```python
from build123d import *

# Parameters (mm, degrees)
SKETCH2_W           = 38.1
SKETCH2_H           = 304.8
SKETCH2_W_2         = 218.44
SKETCH2_H_2         = 38.1
BOSS_EXTRUDE1_DEPTH = 50.8
SKETCH4_W           = 228.6
SKETCH4_H           = 1.6002
CUT_EXTRUDE1_DEPTH  = 5.08


with BuildPart() as part:
    # Sketch2 → Boss-Extrude1 (new body)
    with BuildSketch(Plane(origin=(0, 0, 0), x_dir=(1, 0, 0), z_dir=(0, 1, 0))):
        with Locations((-128.27, 0)):
            Rectangle(SKETCH2_W, SKETCH2_H)
        with Locations((128.27, 0)):
            Rectangle(SKETCH2_W, SKETCH2_H)
        with Locations((0, -133.35)):
            Rectangle(SKETCH2_W_2, SKETCH2_H_2)
        with Locations((0, 133.35)):
            Rectangle(SKETCH2_W_2, SKETCH2_H_2)
    extrude(amount=BOSS_EXTRUDE1_DEPTH)

    # Sketch4 → Cut-Extrude1 (cut)
    with BuildSketch(Plane(origin=(-109.22, 0, 0), x_dir=(0, 0, -1), z_dir=(1, 0, 0))):
        with Locations((0, 37.2999)):
            Rectangle(SKETCH4_W, SKETCH4_H)
    cut_extrude1 = extrude(amount=-CUT_EXTRUDE1_DEPTH, mode=Mode.SUBTRACT)

    # Mirror1: Cut-Extrude1 across plane
    add(cut_extrude1.mirror(Plane(origin=(0, 0, 0), x_dir=(0, 0, 1), z_dir=(1, 0, 0))), mode=Mode.SUBTRACT)


solid = part.part
```
Could you check a few things on this model? Use its own coordinates, in mm. A direction names the side the tool comes from. Round coordinates to 2 decimals unless told otherwise and drop trailing zeros. Loops run counter-clockwise (first coordinate to the right, second up) from the corner with the lowest first, then second, coordinate; pieces in that order, holes last.
Q1. Thinking about a two-plate mould opening in X: for faces 1 (the flat face through (-109.22, 18, 2)), 2 (the flat face through (-133, 0, -2)), 3 (the flat face through (-147.32, 25, 2)), which applies, pulls with the +X half, pulls with the -X half, needs draft (parallel to the pull), parting line crosses it, or undercut?
Q2. On a 3-axis mill with a long thin cutter (end or side, diameter ignored), from which of +Z, -Z, +X, -X, +Y, -Y can I reach the whole of each face in a straight line? I mean faces 4 (the flat face through (-133, 50.8, -2)), 5 (the flat face through (109.22, 44, 2)). Say none if no direction works.
Q3. For P1, Ø5.5, axis at x = -112.5, z = -38.5, coming from the -Y side, with a flat end and sliding along its axis, tell me the tip position at first contact or that it passes through.
Q4. I want a section at A-A (x = 31.5). Write out the boundary of the cut face in (y, z), and give its area (3 significant figures).
Q5. I want a section at B-B (z = -36). Write out the boundary of the cut face in (x, y).
Q6. Please list where these lines run through material, in increasing order: L1, parallel to X at y = 14.5, z = -6; L2, parallel to Z at x = -105, y = 45.5; L3, parallel to Y at x = -110.5, z = 90.5.
Q7. I want a section at C-C (y = 28.5). Write out the boundary of the cut face in (x, z), and give its area (3 significant figures).
Answer below:
1. face 1: undercut
1. face 2: needs draft
1. face 3: pulls with the -X half
2. face 4: +Z, -Z, +X, -X, +Y
2. face 5: +Y, -Y
3. P1: stops at y = 0
4. outline: (0, -152.4) - (50.8, -152.4) - (50.8, -114.3) - (0, -114.3) - close; (0, 114.3) - (50.8, 114.3) - (50.8, 152.4) - (0, 152.4) - close
4. area: 3,870 mm2
5. outline: (-147.32, 0) - (-109.22, 0) - (-109.22, 36.5) - (-114.3, 36.5) - (-114.3, 38.1) - (-109.22, 38.1) - (-109.22, 50.8) - (-147.32, 50.8) - close; (109.22, 0) - (147.32, 0) - (147.32, 50.8) - (109.22, 50.8) - (109.22, 38.1) - (114.3, 38.1) - (114.3, 36.5) - (109.22, 36.5) - close
6. L1: x = -147.32 to -109.22, 109.22 to 147.32
6. L2: z = -152.4 to -114.3, 114.3 to 152.4
6. L3: y = 0 to 36.5, 38.1 to 50.8
7. outline: (-147.32, -152.4) - (147.32, -152.4) - (147.32, 152.4) - (-147.32, 152.4) - close; hole (-109.22, -114.3) - (109.22, -114.3) - (109.22, 114.3) - (-109.22, 114.3) - close
7. area: 39,900 mm2
